Part print with two shaded views. Sizes in mm from the minimum x, y, z corner. Round coordinates to 2 decimals unless told otherwise and drop trailing zeros. Order: outer loops, then holes, each group sorted by start corner. A loop starts at its lowest first (then second) coordinate and runs counter-clockwise, first axis right, second up. Notation, with made-up numbers: (69.5, 70) -> (82.5, 70) arc R14 ccw to (82.5, 82) -> close; hole circle Ø8 at (24, 45). An arc over 180 degrees is marked (long way). Use a Markdown table: item, result. Add a question column.
Item 1: Slice it at D-D, the plane y = 4. State how many separate pieces and enclosed holes the cut face has, plus the area to 3 significant figures.
Item 2: Slice it at B-B, the plane x = 27.5. Give the cut face in (y, z), plus the area to 3 significant figures.
Item 3: Pin check, flat tips, straight feed: pin 1 (5.5 mm diameter, centred on x = 43, z = 62.5, fed in from +Y); pin 2 (2 mm diameter, centred on x = 12, z = 93.5, fed in from +Y). Stop position of each tip, or through.
Item 4: Probe L1, parallel to Z at x = 27.5, y = 2.9; L2, parallel to X at y = 1.1, z = 93.5; L3, parallel to X at y = 0.4, z = 77.5. List the from-to ranges inside material, lowest first.
Item 5: Slice it at A-A, the plane z = 93.5. Give the cut face in (x, y), plus the area to 3 significant figures.
Item 6: Slice it at C-C, the plane z = 20. Give the cut face in (x, y), plus the area to 3 significant figures.
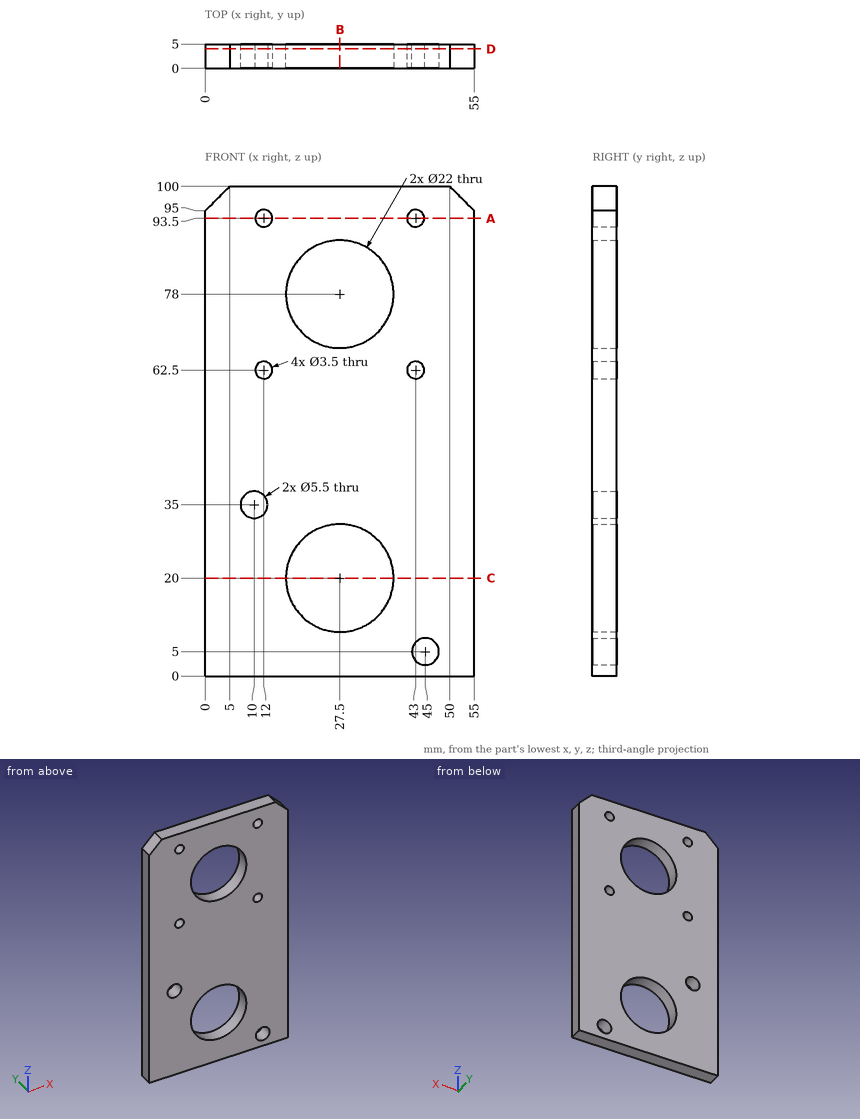
Check sheet entries:
| question | item | result |
|---|---|---|
| 1 | separate pieces | 1 |
| 1 | enclosed holes | 8 |
| 1 | area | 4,630 mm2 |
| 2 | outline | (0, 0) -> (5, 0) -> (5, 9) -> (0, 9) -> close; (0, 31) -> (5, 31) -> (5, 67) -> (0, 67) -> close; (0, 89) -> (5, 89) -> (5, 100) -> (0, 100) -> close |
| 2 | area | 280 mm2 |
| 3 | pin 1 | y = 5 |
| 3 | pin 2 | through |
| 4 | L1 | 0 to 9, 31 to 67, 89 to 100 |
| 4 | L2 | 0 to 10.25, 13.75 to 41.25, 44.75 to 55 |
| 4 | L3 | 0 to 16.51, 38.49 to 55 |
| 5 | outline | (0, 0) -> (10.25, 0) -> (10.25, 5) -> (0, 5) -> close; (13.75, 0) -> (41.25, 0) -> (41.25, 5) -> (13.75, 5) -> close; (44.75, 0) -> (55, 0) -> (55, 5) -> (44.75, 5) -> close |
| 5 | area | 240 mm2 |
| 6 | outline | (0, 0) -> (16.5, 0) -> (16.5, 5) -> (0, 5) -> close; (38.5, 0) -> (55, 0) -> (55, 5) -> (38.5, 5) -> close |
| 6 | area | 165 mm2 |
